Source: CAD feature listing. Evaluate the final solid. Frame: model axes, mm. Coordinates: 2 decimals unless noted, no trailing zeros. Loops run counter-clockwise (first coordinate to the right, second up) from the corner with the lowest first, then second, coordinate; pieces in that order, holes last. Notation, with made-up numbers: (21.25, 29) -> (59.25, 29) arc R27 cw to (59.25, 65) -> close; hole circle Ø3 at (7.25, 16.5). An arc over 180 degrees is marked (long way). One line per question, with ' | ' between items. Start each with the question number.
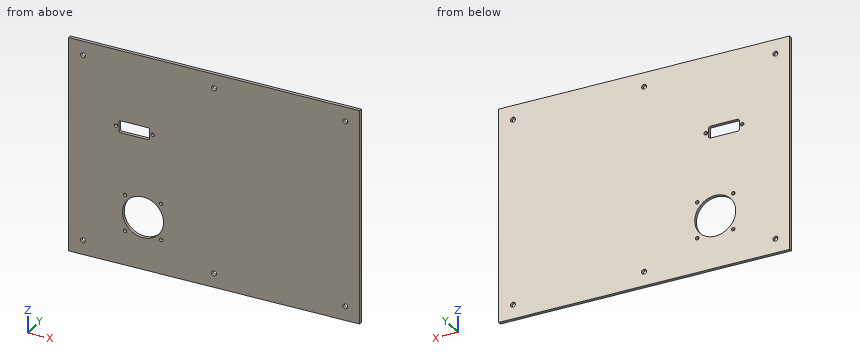
```python
from build123d import *

# Parameters (mm, degrees)
SKETCH_1_W          = 266
SKETCH_1_H          = 196
SKETCH_1_R          = 2.25
EXTRUDE_1_DEPTH     = 3
SKETCH_3_R          = 18.75
SKETCH_3_R_2        = 1.6
CUT_EXTRUDE_1_DEPTH = 4
SKETCH1_R           = 1.6
SKETCH1_W           = 28
SKETCH1_H           = 11
CUT_EXTRUDE1_DEPTH  = 4
FILLET1_R           = 1.5


with BuildPart() as part:
    # Эскиз1 → Бобышка-Вытянуть1 (new body)
    with BuildSketch(Plane(origin=(0, 0, 0), x_dir=(1, 0, 0), z_dir=(0, 1, 0))):
        with Locations((133, 98)):
            Rectangle(SKETCH_1_W, SKETCH_1_H)
        with Locations((13, 183)):
            Circle(SKETCH_1_R, mode=Mode.SUBTRACT)
        with Locations((253, 183)):
            Circle(SKETCH_1_R, mode=Mode.SUBTRACT)
        with Locations((253, 13)):
            Circle(SKETCH_1_R, mode=Mode.SUBTRACT)
        with Locations((13, 13)):
            Circle(SKETCH_1_R, mode=Mode.SUBTRACT)
        with Locations((133, 13)):
            Circle(SKETCH_1_R, mode=Mode.SUBTRACT)
        with Locations((133, 183)):
            Circle(SKETCH_1_R, mode=Mode.SUBTRACT)
    extrude(amount=EXTRUDE_1_DEPTH)

    # Эскиз3 → Вырез-Вытянуть1 (cut, through all)
    with BuildSketch(Plane(origin=(0, 3, 0), x_dir=(1, 0, 0), z_dir=(0, 1, 0))):
        with Locations((68, 148)):
            Circle(SKETCH_3_R)
        with Locations((84.5, 164.5)):
            Circle(SKETCH_3_R_2)
        with Locations((84.5, 131.5)):
            Circle(SKETCH_3_R_2)
        with Locations((51.5, 131.5)):
            Circle(SKETCH_3_R_2)
        with Locations((51.5, 164.5)):
            Circle(SKETCH_3_R_2)
    extrude(amount=-CUT_EXTRUDE_1_DEPTH, mode=Mode.SUBTRACT)

    # Sketch1 → Cut-Extrude1 (cut, through all)
    with BuildSketch(Plane(origin=(0, 3, 0), x_dir=(1, 0, 0), z_dir=(0, 1, 0))):
        with Locations((43.34, 70)):
            Circle(SKETCH1_R)
        with Locations((76.66, 70)):
            Circle(SKETCH1_R)
        with Locations((60, 70)):
            Rectangle(SKETCH1_W, SKETCH1_H)
    extrude(amount=-CUT_EXTRUDE1_DEPTH, mode=Mode.SUBTRACT)

    # Fillet1
    fillet1_edges = [part.edges().sort_by_distance(p)[0] for p in [
        (46, 1.5, -75.5),
        (74, 1.5, -75.5),
        (74, 1.5, -64.5),
        (46, 1.5, -64.5),
    ]]
    fillet(fillet1_edges, radius=FILLET1_R)


solid = part.part
```
(1) Cut plane B-B, the plane z = -153. Return the cut outline in (x, y).
(2) Cut plane A-A, the plane y = 1. State how many separate pieces and enclosed holes the cut face has, and give its area (3 significant figures).
(3) Ray query, L1, parallel to X at y = 2, z = -70; L2, parallel to X at y = 1.9, z = -13; L3, parallel to Z at x = 133, y = 1.35. Return the intervals inside material, ascending.
Here are the results:
1) outline: (0, 0) -> (49.93, 0) -> (49.93, 3) -> (0, 3) -> close; (86.07, 0) -> (266, 0) -> (266, 3) -> (86.07, 3) -> close
2) separate pieces: 1 | enclosed holes: 14 | area: 50,600 mm2
3) L1: x = 0 to 41.74, 44.94 to 46, 74 to 75.06, 78.26 to 266 | L2: x = 0 to 10.75, 15.25 to 130.75, 135.25 to 250.75, 255.25 to 266 | L3: z = -196 to -185.25, -180.75 to -15.25, -10.75 to 0
